The model under review builds one solid part; all positions refer to its coordinate system, in mm. Coordinates: 2 decimals unless noted, no trailing zeros. Loops run counter-clockwise (first coordinate to the right, second up) from the corner with the lowest first, then second, coordinate; pieces in that order, holes last. Notation, with made-up numbers: (49.25, 74) - (104.25, 74) arc R29 cw to (104.25, 105) - close; hole circle Ø9 at (52, -16). An arc over 180 degrees is marked (long way). Answer in a Markdown table with one row per item. Add a question column.
(1) For P1, Ø1, axis at x = -170, y = 1, coming from the +Z side; P2, Ø1.6, axis at x = 170, y = 2, coming from the -Z side; P3, Ø1, axis at y = 2.5, z = 19.5, coming from the +X side, all flat-tipped, find the tip position at first contact; note any pin that passes through.
(2) For line 1 along X through (y, z) = (1.6, 0); line 2 along Z through (x, y) = (-146.5, 0.7); line 3 along X through (y, z) = (1.45, 16), list the stretches that pass through material, from the lowest coordinate up.
(3) We need section B-B on z = 22. Write out the cut boundary in (x, y) (3 decimals).
(4) We need section A-A on y = 1.3. Write out the cut boundary in (x, z).
from build123d import *

# Parameters (mm, degrees)
SKETCH1_W           = 333
SKETCH1_H           = 50
SKETCH1_R           = 1.9
SKETCH1_W_2         = 6.35
SKETCH1_H_2         = 10
BOSS_EXTRUDE1_DEPTH = 3.175


with BuildPart() as part:
    # Sketch1 → Boss-Extrude1 (new body)
    with BuildSketch(Plane(origin=(0, 0, 0), x_dir=(1, 0, 0), z_dir=(0, 1, 0))):
        Rectangle(SKETCH1_W, SKETCH1_H)
        Circle(SKETCH1_R, mode=Mode.SUBTRACT)
        with Locations((50, 0)):
            Circle(SKETCH1_R, mode=Mode.SUBTRACT)
        with Locations((-50, 0)):
            Circle(SKETCH1_R, mode=Mode.SUBTRACT)
        with Locations((146.5, 0)):
            Circle(SKETCH1_R, mode=Mode.SUBTRACT)
        with Locations((-146.5, 0)):
            Circle(SKETCH1_R, mode=Mode.SUBTRACT)
        with Locations((-169.675, 10)):
            Rectangle(SKETCH1_W_2, SKETCH1_H_2)
        with Locations((169.675, 10)):
            Rectangle(SKETCH1_W_2, SKETCH1_H_2)
        with Locations((169.675, -10)):
            Rectangle(SKETCH1_W_2, SKETCH1_H_2)
        with Locations((-169.675, -10)):
            Rectangle(SKETCH1_W_2, SKETCH1_H_2)
    extrude(amount=BOSS_EXTRUDE1_DEPTH)


solid = part.part
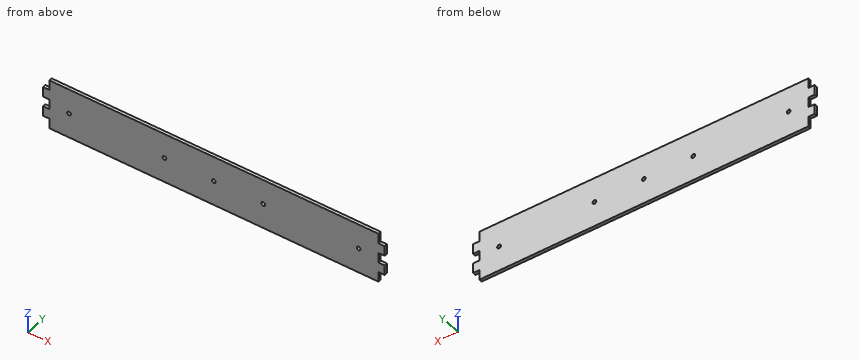
Outcome:
| question | item | result |
|---|---|---|
| 1 | P1 | z = 15 |
| 1 | P2 | z = -15 |
| 1 | P3 | x = 166.5 |
| 2 | line 1 | -166.5 to -148.4, -144.6 to -51.9, -48.1 to -1.9, 1.9 to 48.1, 51.9 to 144.6, 148.4 to 166.5 |
| 2 | line 2 | -25 to -1.9, 1.9 to 25 |
| 2 | line 3 | -166.5 to 166.5 |
| 3 | outline | (-166.5, 0) - (166.5, 0) - (166.5, 3.175) - (-166.5, 3.175) - close |
| 4 | outline | (-172.85, -15) - (-166.5, -15) - (-166.5, -25) - (166.5, -25) - (166.5, -15) - (172.85, -15) - (172.85, -5) - (166.5, -5) - (166.5, 5) - (172.85, 5) - (172.85, 15) - (166.5, 15) - (166.5, 25) - (-166.5, 25) - (-166.5, 15) - (-172.85, 15) - (-172.85, 5) - (-166.5, 5) - (-166.5, -5) - (-172.85, -5) - close; hole circle Ø3.8 at (-146.5, 0); hole circle Ø3.8 at (-50, 0); hole circle Ø3.8 at (0, 0); hole circle Ø3.8 at (50, 0); hole circle Ø3.8 at (146.5, 0) |
